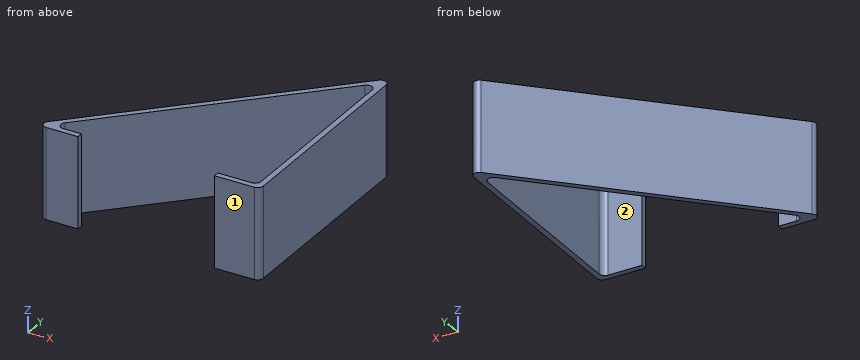
Autodesk Inventor part; units mm, degrees
ref_plane "YZ Plane" through (0, 0, 0) normal (1, 0, 0) x (0, 1, 0)
ref_plane "XZ Plane" through (0, 0, 0) normal (0, 1, 0) x (-1, 0, 0)
ref_plane "XY Plane" through (0, 0, 0) normal (0, 0, 1) x (1, 0, 0)
sketch "Sketch1" plane through (0, 0, 0) normal (0, 0, 1) x (1, 0, 0)
  line L0 (0, 0) -> (25.4, 0)
  line L1 (0, 0) -> (127, 127)
  line L2 (127, 127) -> (127, 0)
  line L3 (123.825, 3.175) -> (123.825, 119.3349)
  line L4 (123.825, 119.3349) -> (7.6651, 3.175)
  line L5 (7.6651, 3.175) -> (25.4, 3.175)
  line L6 (25.4, 3.175) -> (25.4, 0)
  line L7 (127, 0) -> (101.6, 0)
  line L8 (101.6, 0) -> (101.6, 3.175)
  line L9 (127, 3.175) -> (127, 0)
  line L10 (101.6, 3.175) -> (123.825, 3.175)
  dimension "d0" = 127
  dimension "d1" = 127
  dimension "d2" = 25.4
  dimension "d4" = 3.175
  dimension "d5" = 3.175
  dimension "d6" = 3.175
  dimension "d7" = 25.4
  dimension "d8" = 3.175
extrude "Extrusion1" add sketch "Sketch1" along normal blind 50.8
fillet "Fillet1" radius 3.175 6 edges at (7.6651, 3.175, 25.4) (123.825, 119.3349, 25.4) (123.825, 3.175, 25.4) (127, 0, 25.4) (127, 127, 25.4) (0, 0, 25.4)
equation "\"d5\" = d4"
equation "\"d6\" = d5"
equation "\"d8\" = d5"
properties part number "apendage polycarb wedge"
Geometry: final body of the model. Coordinates: model frame, mm. Face numbers are marked on the shaded views. A direction names the side the tool comes from. Give positions to 0.01 mm unless a question says otherwise; leave off trailing zeros. Loops run counter-clockwise (first coordinate to the right, second up) from the corner with the lowest first, then second, coordinate; pieces in that order, holes last. Notation, with made-up numbers: M 32.5,-32.75 L 57.5,-32.75 A19 ccw 57.5,-5.75 Z; hole C 86.25,10 d11. An arc over 180 degrees is marked long. Put each result on its own line as item: value.
1) Reachability of the marked faces 1 and 2 from +Z, -Z, +X, -X, +Y, -Y: full face, straight path, thin tool, end or side. Return the list, or none.
Computed values:
face 1: +Z, -Z, +X, -X, -Y
face 2: +Z, -Z
2) Cut plane A-A, the plane z = 12. Return the cut outline in (x, y) (1 decimal).
Computed values:
outline: M 5.4,5.4 A3.2 ccw 7.7,0 L 25.4,0 L 25.4,3.2 L 15.3,3.2 A3.2 cw 13.1,8.6 L 118.4,113.9 A3.2 cw 123.8,111.7 L 123.8,6.3 A3.2 cw 120.7,3.2 L 101.6,3.2 L 101.6,0 L 123.8,0 A3.2 ccw 127,3.2 L 127,119.3 A3.2 ccw 121.6,121.6 Z
3) First-contact query: P1, Ø5.5, axis at x = 107.5, z = 20, coming from the +Y side; P2, Ø6, axis at x = 68.5, z = 28.5, coming from the +Y side; P3, Ø3, axis at x = 18.5, z = 14.5, coming from the +Y side. Flat tips, straight axial feed; report the tip coordinate or a pass-through.
Computed values:
P1: stops at y = 110.25
P2: stops at y = 71.5
P3: stops at y = 20
4) Cut plane B-B, the plane x = 116. Return the cut outline in (y, z) (3 decimals), plus the area to 3 significant figures.
Computed values:
outline: M 0,0 L 3.175,0 L 3.175,50.8 L 0,50.8 Z; M 111.51,0 L 116,0 L 116,50.8 L 111.51,50.8 Z
area: 389 mm^2
5) Cut plane C-C, the plane y = 55. Return the cut outline in (x, z) (3 decimals), plus the area to 3 significant figures.
Computed values:
outline: M 55,0 L 59.49,0 L 59.49,50.8 L 55,50.8 Z; M 123.825,0 L 127,0 L 127,50.8 L 123.825,50.8 Z
area: 389 mm^2
6) Cut plane D-D, the plane x = 56. Return the cut outline in (y, z), plus the area to 3 significant figures.
Computed values:
outline: M 51.51,0 L 56,0 L 56,50.8 L 51.51,50.8 Z
area: 228 mm^2
7) Material intervals for L1, parallel to X at y = 68, z = 24 (3 decimals); L2, parallel to X at y = 102, z = 16.5 (3 decimals); L3, parallel to Y at x = 118, z = 11.5 (3 decimals), sorted ascending. Write a range as from..to.
Computed values:
L1: x = 68..72.49, 123.825..127
L2: x = 102..106.49, 123.825..127
L3: y = 0..3.175, 113.51..118
